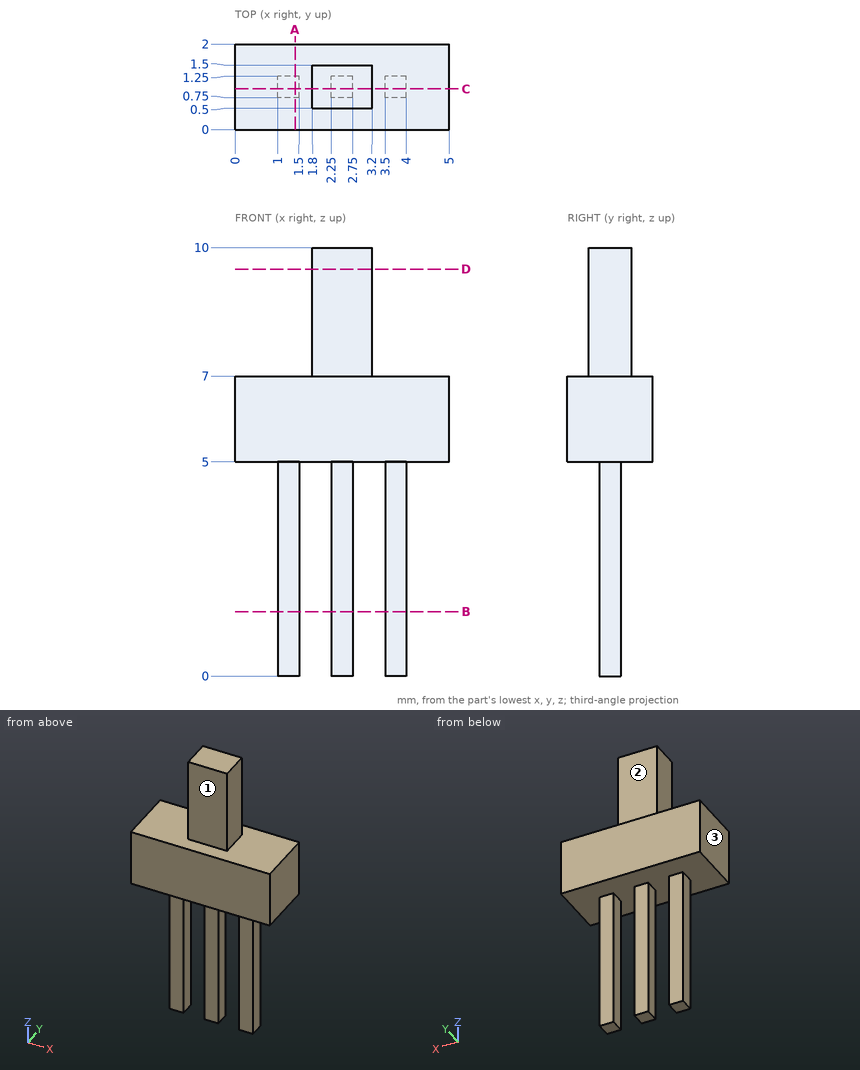
Could you check a few things on this drawing? It's one solid part, dimensions in mm from its lowest x, y, z. A direction names the side the tool comes from. Give positions to 0.01 mm unless a question says otherwise; leave off trailing zeros. Loops run counter-clockwise (first coordinate to the right, second up) from the corner with the lowest first, then second, coordinate; pieces in that order, holes last. Notation, with made-up numbers: (-19, -34) -> (-14, -34) arc R15 ccw to (-14, -29) -> close; hole circle Ø8 at (1, 23.25). An arc over 180 degrees is marked (long way). Answer as CSV lines item,"result". Start each with the question number.
(1) Which directions (+Z, -Z, +X, -X, +Y, -Y) give clear straight access to the entire face, cutting with the end or side of a thin tool? Please do the marked faces 1, 2 and 3.
(2) If we section it at B-B on z = 1.5: Write out the boundary of the cut face in (x, y), then the cut area to 3 significant figures.
(3) I need wall thicknesses on probe 1 along X at (y, z) = (0.9, 4.25); probe 2 along Z at (x, y) = (0.8, 0.95); probe 3 along X at (y, z) = (0.55, 8.5). Which ranges of each line are inside material? Lowest first, please.
(4) If we section it at C-C on y = 0.95: Write out the boundary of the cut face in (x, z).
(5) If we section it at D-D on z = 9.5: Write out the boundary of the cut face in (x, y).
(6) If we section it at A-A on x = 1.4: Write out the boundary of the cut face in (y, z), then the cut area to 3 significant figures.
(7) I'm going to push flat-ended pins straight in: pin 1 Ø2 at (x, z) = (4.5, 4.5) entering from -Y; pin 2 Ø1.5 at (x, z) = (2.5, 9) entering from +Y; pin 3 Ø0.6 at (x, z) = (1, 2) entering from +Y; pin 4 Ø0.6 at (x, z) = (4, 3) entering from -Y. Where does each tip first touch, or does it pass through?
Computed:
1,face 1,"+Z, +X, -X, -Y"
1,face 2,"+Z, +X, -X, +Y"
1,face 3,"+Z, -Z, -X, +Y, -Y"
2,outline,"(1, 0.75) -> (1.5, 0.75) -> (1.5, 1.25) -> (1, 1.25) -> close; (2.25, 0.75) -> (2.75, 0.75) -> (2.75, 1.25) -> (2.25, 1.25) -> close; (3.5, 0.75) -> (4, 0.75) -> (4, 1.25) -> (3.5, 1.25) -> close"
2,area,"0.750 mm2"
3,probe 1,"x = 1 to 1.5, 2.25 to 2.75, 3.5 to 4"
3,probe 2,"z = 5 to 7"
3,probe 3,"x = 1.8 to 3.2"
4,outline,"(0, 5) -> (1, 5) -> (1, 0) -> (1.5, 0) -> (1.5, 5) -> (2.25, 5) -> (2.25, 0) -> (2.75, 0) -> (2.75, 5) -> (3.5, 5) -> (3.5, 0) -> (4, 0) -> (4, 5) -> (5, 5) -> (5, 7) -> (3.2, 7) -> (3.2, 10) -> (1.8, 10) -> (1.8, 7) -> (0, 7) -> close"
5,outline,"(1.8, 0.5) -> (3.2, 0.5) -> (3.2, 1.5) -> (1.8, 1.5) -> close"
6,outline,"(0, 5) -> (0.75, 5) -> (0.75, 0) -> (1.25, 0) -> (1.25, 5) -> (2, 5) -> (2, 7) -> (0, 7) -> close"
6,area,"6.50 mm2"
7,pin 1,"stops at y = 0"
7,pin 2,"stops at y = 1.5"
7,pin 3,"stops at y = 1.25"
7,pin 4,"stops at y = 0.75"
